Geometry: final body of the model. Coordinates: model frame, mm. A direction names the side the tool comes from. Give positions to 0.01 mm unless a question says otherwise; leave off trailing zeros. Write each loop counter-clockwise with the first axis right and the second up, starting at its lowest first coordinate (ties: lowest second). Pieces come first, ordered by that corner, then holes. Notation, with made-up numbers: M 37.5,-35 L 66.5,-35 A12 cw 66.5,-31 Z; hole C -5,-37 d1. An arc over 180 degrees is marked long. Use a Markdown table: item, result. Add a question column.
(1) Reachability of faces 1 (the cylindrical face through (-0.59, 4.46, 30.97)), 2 (the cylindrical face through (-5.37, -1.19, 7.75)) from +Z, -Z, +X, -X, +Y, -Y: full face, straight path, thin tool, end or side. Return the list, or none.
(2) Pin query (flat end, axial travel): pin 1 Ø3 at (y, z) = (2, -22) entering from +X; pin 2 Ø1 at (x, y) = (-4, 4) entering from +Z; pin 3 Ø4 at (y, z) = (4, 20.5) entering from +X. Return the tip coordinate at first contact, or that it passes through.
(3) Material intervals for L1, parallel to X at y = 0, z = -20.75 (3 decimals); L2, parallel to X at y = 0, z = -23 (3 decimals); L3, parallel to Y at x = 0.25, z = 30, sorted ascending.
(4) Cut plane A-A (z = -18). Output: boundary loops of the cut face in (x, y) (3 decimals), plus the area to 3 significant figures.
(5) Draft query along X for faces 3 (the cylindrical face through (4.72, 1.49, 34.87)), 4 (the flat face through (-1.475, 0, -22)). Return one class per face: released by +X, released by -X, zero draft, split by the parting line, or undercut.
```python
from build123d import *

# Parameters (mm, degrees)
CUT_EXTRUDE1_DEPTH  = 14
SKETCH5_R           = 4.5
BOSS_EXTRUDE1_DEPTH = 4
SKETCH6_R           = 4.95
BOSS_EXTRUDE2_DEPTH = 4
CHAMFER1_SIZE       = 0.2


with BuildPart() as part:
    # Sketch2 → Revolve2 (revolve)
    with BuildSketch(Plane(origin=(0, 0, 0), x_dir=(0, 0, -1), z_dir=(1, 0, 0))):
        Polygon((-29, 0), (29, 0), (29, 5.5), (26.5, 5.5), (26.5, 5.25), (25, 5.25), (25, 5.5), (21.35, 5.5), (21.35, 5.25), (19.85, 5.25), (19.85, 5.5), (16.2, 5.5), (16.2, 5.25), (14.7, 5.25), (14.7, 5.5), (11.05, 5.5), (11.05, 5.25), (9.55, 5.25), (9.55, 5.5), (5.9, 5.5), (5.9, 5.25), (4.4, 5.25), (4.4, 5.5), (0.75, 5.5), (0.75, 5.25), (-0.75, 5.25), (-0.75, 5.5), (-4.4, 5.5), (-4.4, 5.25), (-5.9, 5.25), (-5.9, 5.5), (-9.55, 5.5), (-9.55, 5.25), (-11.05, 5.25), (-11.05, 5.5), (-14.7, 5.5), (-14.7, 5.25), (-16.2, 5.25), (-16.2, 5.5), (-19.85, 5.5), (-19.85, 5.25), (-21.35, 5.25), (-21.35, 5.5), (-25, 5.5), (-25, 5.25), (-26.5, 5.25), (-26.5, 5.5), (-29, 5.5), align=None)
    revolve(axis=Axis((0, 0, -29), (0, 0, -1)))

    # Sketch3 → Cut-Extrude1 (cut)
    with BuildSketch(Plane(origin=(0, 0, -29), x_dir=(-1, 0, 0), z_dir=(0, 0, -1))):
        with BuildLine():
            Line((1.475, 1.529705854), (1.475, -1.529705854))
            ThreePointArc((1.475, -1.529705854), (-2.125, 0), (1.475, 1.529705854))
        make_face()
    extrude(amount=-CUT_EXTRUDE1_DEPTH, mode=Mode.SUBTRACT)

    # Sketch5 → Boss-Extrude1 (add)
    with BuildSketch(Plane.XY.offset(29)):
        Circle(SKETCH5_R)
    extrude(amount=BOSS_EXTRUDE1_DEPTH)

    # Sketch6 → Boss-Extrude2 (add)
    with BuildSketch(Plane.XY.offset(33)):
        Circle(SKETCH6_R)
    extrude(amount=BOSS_EXTRUDE2_DEPTH)

    # Chamfer1
    chamfer1_edges = [part.edges().sort_by_distance(p)[0] for p in [
        (-4.5, 0, 29),
        (-4.5, 0, 33),
        (-4.95, 0, 37),
        (0, -5.25, -26.5),
        (0, -5.25, -25),
        (0, -5.25, -21.35),
        (0, -5.25, -19.85),
        (0, -5.25, -16.2),
        (0, -5.25, -14.7),
        (0, -5.25, -11.05),
        (0, -5.25, -9.55),
        (0, -5.25, -5.9),
        (0, -5.25, -4.4),
        (0, -5.25, -0.75),
        (0, -5.25, 0.75),
        (0, -5.25, 4.4),
        (0, -5.25, 5.9),
        (0, -5.25, 9.55),
        (0, -5.25, 11.05),
        (0, -5.25, 14.7),
        (0, -5.25, 16.2),
        (0, -5.25, 19.85),
        (0, -5.25, 21.35),
        (0, -5.25, 25),
        (0, -5.25, 26.5),
    ]]
    chamfer(chamfer1_edges, length=CHAMFER1_SIZE)


solid = part.part
```
Answer list:
| question | item | result |
|---|---|---|
| 1 | face 1 | none |
| 1 | face 2 | +Z, -Z |
| 2 | pin 1 | x = 5.48 |
| 2 | pin 2 | z = 29 |
| 2 | pin 3 | x = 5.08 |
| 3 | L1 | -5.25 to -1.475, 2.125 to 5.25 |
| 3 | L2 | -5.5 to -1.475, 2.125 to 5.5 |
| 3 | L3 | -4.49 to 4.49 |
| 4 | outline | C 0,0 d11; hole M -1.475,-1.53 A2.125 ccw long -1.475,1.53 Z |
| 4 | area | 82.2 mm² |
| 5 | face 3 | split by the parting line |
| 5 | face 4 | undercut |
